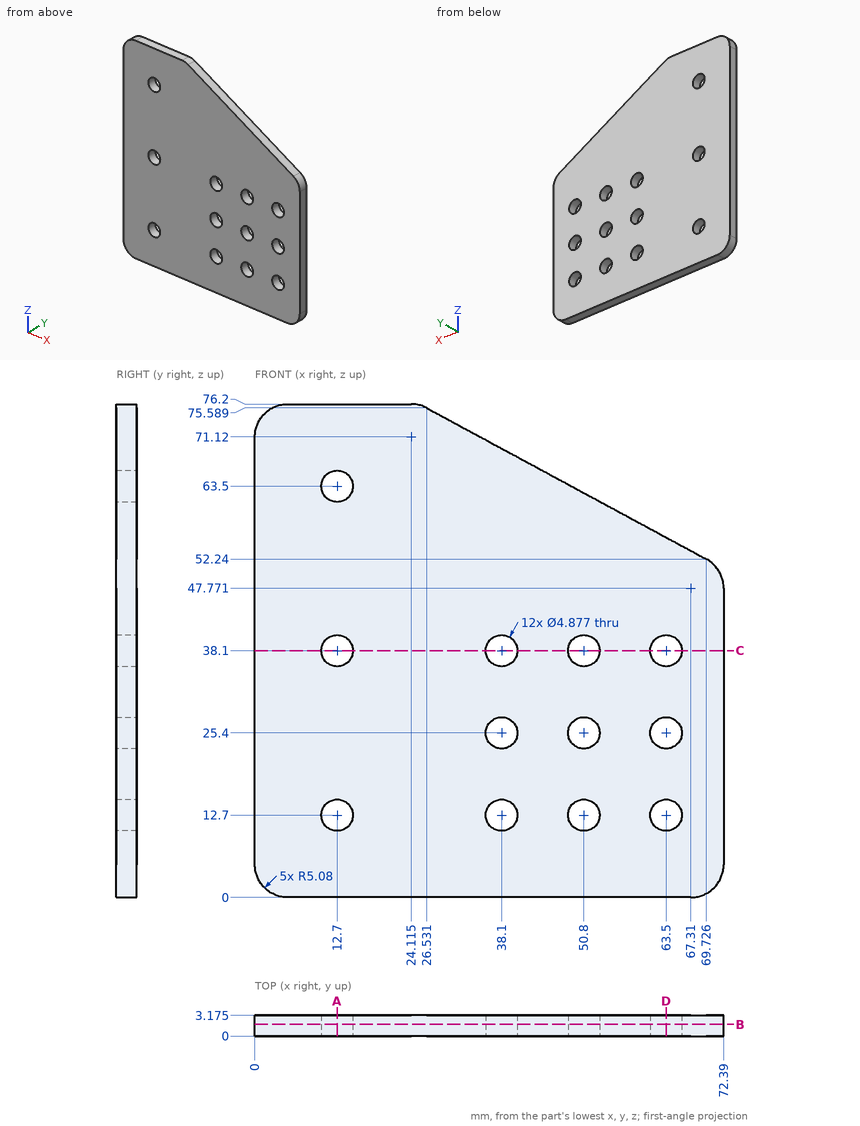
Design review of the part shown in the three views and the two pictorial views. Dimensions are in mm from the part's minimum x, y and z. Coordinates: 2 decimals unless noted, no trailing zeros. Loops run counter-clockwise (first coordinate to the right, second up) from the corner with the lowest first, then second, coordinate; pieces in that order, holes last. Notation, with made-up numbers: (2, 74) -> (7, 74) arc R18 cw to (7, 96) -> close; hole circle Ø6 at (83, -25). An arc over 180 degrees is marked (long way). Answer as CSV lines item,"result".
Item 1: For L1, parallel to X at y = 1.9, z = 12.7; L2, parallel to X at y = 1.1, z = 25.4; L3, parallel to X at y = 2.85, z = 63 (1 decimal), list the stretches that pass through material, from the lowest coordinate up.
Results below:
L1,"x = 0 to 10.26, 15.14 to 35.66, 40.54 to 48.36, 53.24 to 61.06, 65.94 to 72.39"
L2,"x = 0 to 35.66, 40.54 to 48.36, 53.24 to 61.06, 65.94 to 72.39"
L3,"x = 0 to 10.3, 15.1 to 49.8"
Item 2: Take a section at C-C, the plane z = 38.1. State the section outline as (x, y) points (1 decimal).
Results below:
outline,"(0, 0) -> (10.3, 0) -> (10.3, 3.2) -> (0, 3.2) -> close; (15.1, 0) -> (35.7, 0) -> (35.7, 3.2) -> (15.1, 3.2) -> close; (40.5, 0) -> (48.4, 0) -> (48.4, 3.2) -> (40.5, 3.2) -> close; (53.2, 0) -> (61.1, 0) -> (61.1, 3.2) -> (53.2, 3.2) -> close; (65.9, 0) -> (72.4, 0) -> (72.4, 3.2) -> (65.9, 3.2) -> close"
Item 3: Take a section at A-A, the plane x = 12.7. State the section outline as (y, z) points (1 decimal).
Results below:
outline,"(0, 0) -> (3.2, 0) -> (3.2, 10.3) -> (0, 10.3) -> close; (0, 15.1) -> (3.2, 15.1) -> (3.2, 35.7) -> (0, 35.7) -> close; (0, 40.5) -> (3.2, 40.5) -> (3.2, 61.1) -> (0, 61.1) -> close; (0, 65.9) -> (3.2, 65.9) -> (3.2, 76.2) -> (0, 76.2) -> close"
Item 4: Take a section at D-D, the plane x = 63.5. State the section outline as (y, z) points (1 decimal), and give its area (3 significant figures).
Results below:
outline,"(0, 0) -> (3.2, 0) -> (3.2, 10.3) -> (0, 10.3) -> close; (0, 15.1) -> (3.2, 15.1) -> (3.2, 23) -> (0, 23) -> close; (0, 27.8) -> (3.2, 27.8) -> (3.2, 35.7) -> (0, 35.7) -> close; (0, 40.5) -> (3.2, 40.5) -> (3.2, 55.6) -> (0, 55.6) -> close"
area,"130 mm2"
Item 5: Take a section at B-B, the plane y = 1.8. Count the separate pieces of the cut face and the enclosed holes in it, and give its area (3 significant figures).
Results below:
separate pieces,"1"
enclosed holes,"12"
area,"4,680 mm2"
